from build123d import *

# Parameters (mm, degrees)
F0_R            = 125
F1_DEPTH        = 3
F2_R            = 1.5
F3_DEPTH        = 6.001
F5_R            = 29
F6_DEPTH        = 6.001
F6_COPIES_COUNT = 8
F5_R_2          = 30
F7_DEPTH        = 3
F7_COPIES_COUNT = 8
F9_DEPTH        = 6.001


# Not quite as in the source:
# - a pattern or mirror of a feature is missing from the dataset's text; its kind, count and spacing are read off the source's solid


with BuildPart() as f1:
    # F0 (on Top) → F1 (new body, symmetric)
    with BuildSketch(Plane.XY):
        Circle(F0_R)
    extrude(amount=F1_DEPTH, both=True)

    # F2 (on face) → F3 (cut, through all)
    with BuildSketch(Plane(origin=(0, 0, -3), x_dir=(1, 0, 0), z_dir=(0, 0, -1))):
        Circle(F2_R)
    extrude(amount=-F3_DEPTH, mode=Mode.SUBTRACT)

    # F5 (on face) → F6 (cut, through all)
    with BuildSketch(Plane.XY.offset(3)):
        with Locations((83.46965909, 0)):
            Circle(F5_R)
    f6 = extrude(amount=-F6_DEPTH, mode=Mode.SUBTRACT)

    # F6_copies: F6 ×8 about axis
    f6_copies_axis = Axis((0, 0, 0), (0, 0, 1))
    for i in range(1, F6_COPIES_COUNT):
        add(f6.rotate(f6_copies_axis, i * 360 / F6_COPIES_COUNT), mode=Mode.SUBTRACT)

    # F5 (on face) → F7 (cut)
    with BuildSketch(Plane.XY.offset(3)):
        with Locations((83.46965909, 0)):
            Circle(F5_R_2)
        with Locations((83.46965909, 0)):
            Circle(F5_R, mode=Mode.SUBTRACT)
    f7 = extrude(amount=-F7_DEPTH, mode=Mode.SUBTRACT)

    # F7_copies: F7 ×8 about axis
    f7_copies_axis = Axis((0, 0, 0), (0, 0, 1))
    for i in range(1, F7_COPIES_COUNT):
        add(f7.rotate(f7_copies_axis, i * 360 / F7_COPIES_COUNT), mode=Mode.SUBTRACT)

    # F8 (on face) → F9 (cut, through all)
    with BuildSketch(Plane.XY.offset(3)):
        with BuildLine():
            add(Edge.make_bspline(
                [(-44.3258620799, -15.0524862111), (-48.3588050122, -20.1152564211), (-23.0924792953, -39.7830257512), (5.512565217, -41.0118510348), (16.0001607542, -11.0681310793), (-38.9619666275, -8.3188997057), (-44.3258620799, -15.0524862111)],
                knots=[0, 0, 0, 0, 0.2444791319, 0.4878585615, 0.6748378229, 1, 1, 1, 1], degree=3))
        make_face()
        with BuildLine():
            add(Edge.make_bspline(
                [(-45.671308504, 13.8018518265), (-46.0710162563, 7.3414722241), (-14.0930848504, 5.7227478351), (10.0436210659, 21.123332585), (1.4595442067, 51.6672296743), (-45.1396891305, 22.3942870163), (-45.671308504, 13.8018518265)],
                knots=[0, 0, 0, 0, 0.2444791319, 0.4878585615, 0.6748378229, 1, 1, 1, 1], degree=3))
        make_face()
        with BuildLine():
            add(Edge.make_bspline(
                [(19.5642778018, -27.1424591751), (25.1230293593, -30.4585641219), (41.2175010078, -2.7786734428), (38.591626534, 25.7320853401), (7.5102643018, 32.1011470227), (12.1710260995, -22.7319727037), (19.5642778018, -27.1424591751)],
                knots=[0, 0, 0, 0, 0.2444791319, 0.4878585615, 0.6748378229, 1, 1, 1, 1], degree=3))
        make_face()
    extrude(amount=-F9_DEPTH, mode=Mode.SUBTRACT)


solid = f1.part
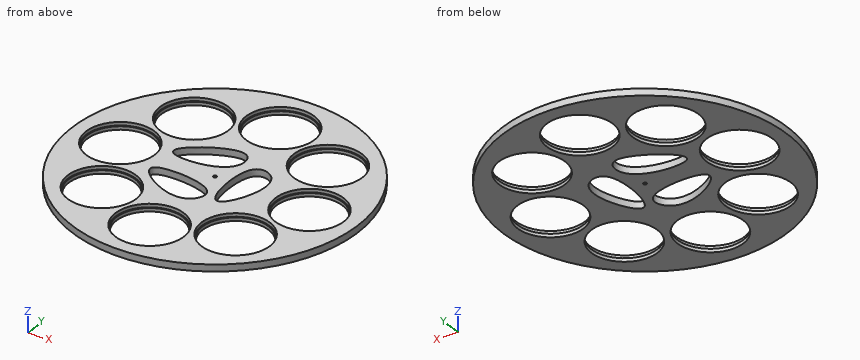
Check sheet for the modelled part. Datum: model origin and axes. Units: mm. Coordinates: 2 decimals unless noted, no trailing zeros. Loops run counter-clockwise (first coordinate to the right, second up) from the corner with the lowest first, then second, coordinate; pieces in that order, holes last. Notation, with made-up numbers: (52, -3) -> (108, -3) arc R21 cw to (108, 23) -> close; hole circle Ø1 at (66.5, 36.5). An arc over 180 degrees is marked (long way). Answer in a Markdown table with one row per item.
1. Sectioned sample at C-C, the plane y = -23. Give the number of separate pieces and of enclosed holes in the cut face, then the cut area to 3 significant figures.
Check values:
| item | result |
|---|---|
| separate pieces | 5 |
| enclosed holes | 0 |
| area | 658 mm2 |
2. Material ranges on line 1 along X through (y, z) = (1, 2.5); line 2 along Y through (x, z) = (84.5, -2.5); line 3 along Y through (x, z) = (9.5, -0.25), recorded low to high. Write a range as [from, to].
Check values:
| item | result |
|---|---|
| line 1 | x = [-125, -113.45], [-53.49, -1.12], [1.12, 12.33], [38.06, 53.49], [113.45, 125] |
| line 2 | y = [-92.11, -72.87], [-45.17, -28.98], [28.98, 45.17], [72.87, 92.11] |
| line 3 | y = [-124.64, -110.87], [-56.07, 56.07], [110.87, 124.64] |
3. Sectioned sample at A-A, the plane x = 97.5. Record the boundary of the cut face in (y, z).
Check values:
| item | result |
|---|---|
| outline | (-78.22, -3) -> (-25.38, -3) -> (-25.38, 0) -> (-26.52, 0) -> (-26.52, 3) -> (-78.22, 3) -> close; (25.38, -3) -> (78.22, -3) -> (78.22, 3) -> (26.52, 3) -> (26.52, 0) -> (25.38, 0) -> close |
4. Sectioned sample at B-B, the plane y = -104.5. Record the boundary of the cut face in (x, z), then the cut area to 3 significant figures.
Check values:
| item | result |
|---|---|
| outline | (-68.59, -3) -> (-19.97, -3) -> (-19.97, 0) -> (-21.39, 0) -> (-21.39, 3) -> (-68.59, 3) -> close; (19.97, -3) -> (68.59, -3) -> (68.59, 3) -> (21.39, 3) -> (21.39, 0) -> (19.97, 0) -> close |
| area | 575 mm2 |
5. Go/stop test with flat-tipped pins: pin 1 (1.5 mm diameter, centred on y = 25.5, z = -2, fed in from -X); pin 2 (2 mm diameter, centred on x = 43.5, z = 0, fed in from +Y); pin 3 (1.5 mm diameter, centred on x = -52, z = -1, fed in from -Y). Record where each tip stops, or that it passes through.
Check values:
| item | result |
|---|---|
| pin 1 | stops at x = -122.53 |
| pin 2 | stops at y = 117.55 |
| pin 3 | stops at y = -114.01 |
